Geometry check sheet. Reference: the model listing, model coordinates, mm. A direction names the side the tool comes from. Coordinates: 2 decimals unless noted, no trailing zeros. Order: outer loops, then holes, each group sorted by start corner. A loop starts at its lowest first (then second) coordinate and runs counter-clockwise, first axis right, second up. Notation, with made-up numbers: (8.5, -35.75) - (49.5, -35.75) arc R22 cw to (49.5, -13.75) - close; hole circle Ø11 at (75.5, -6.75). An arc over 180 degrees is marked (long way). Return JSON: item names as keys, results as strings. Group by question number.
Item 1: Section check C-C on y = 10. Enter the section's corners in (x, z) (3 decimals).
Item 2: Draft check along X on faces 1 (the flat face through (6, -14, 6.35)), 2 (the flat face through (6, -16.5, 3)), 3 (the cylindrical face through (-0.08, -32.25, 6.37)), 4 (the flat face through (9.157, 15.049, 3.87)). Enter one of: pulls with the +X half, pulls with the -X half, needs draft (parallel to the pull), parting line crosses it, or undercut.
Item 3: Gauge pin test, flat ends, axial feed: pin 1 (1.5 mm diameter, centred on y = -5.5, z = 2, fed in from +X) (3 decimals); pin 2 (1.9 mm diameter, centred on x = -4, y = -15, fed in from -Z) (3 decimals); pin 3 (1.5 mm diameter, centred on y = -14.5, z = 4, fed in from -X); pin 4 (8.5 mm diameter, centred on x = -2, y = -28.5, fed in from -Z). Record the tip position at first contact, or that the pin passes through.
Item 4: Section check D-D on y = -15. Enter the section's corners in (x, z) (3 decimals), then the cut area to 3 significant figures.
Item 5: Scan lines: probe 1 along Y at (x, z) = (7, 7.5); probe 2 along Y at (x, z) = (-4, 6); probe 3 along Y at (x, z) = (-1.75, 7). Record each from-to range of solid material in increasing order.
Item 6: Tool access check on faces 5 (the flat face through (6, 14, 6.35)), 6 (the flat face through (9, 11.5, 3)), 7 (the flat face through (1, -19.806, 6)), 8 (the flat face through (-1, -24, 4.85)), 9 (the flat face through (-6.641, -21, 6)). Record the directions out of +Z, -Z, +X, -X, +Y, -Y that give a thin tool (end or side, any length) a straight path to the whole face; none if there is none.
Item 7: Section check A-A on y = -8. Enter the section's corners in (x, z) (3 decimals), then the cut area to 3 significant figures.
Item 8: Section check B-B on x = 2.25. Enter the section's corners in (y, z).
from build123d import *

# Parameters (mm, degrees)
PAD_DEPTH       = 6.35
SKETCH001_W     = 19.26
SKETCH001_H     = 23
PAD001_DEPTH    = 1.5
SKETCH003_R     = 1.58
POCKET_DEPTH    = 98.88341
SKETCH002_W     = 4.4
SKETCH002_H     = 3.6
POCKET001_DEPTH = 14.106
FILLET_R        = 7
FILLET001_R     = 0.5
SKETCH004_R     = 1.58
PAD002_DEPTH    = 3


with BuildPart() as part:
    # Sketch → Pad (new body)
    with BuildSketch(Plane.XY):
        Polygon((4.355, -11.5), (-12.105, -11.5), (-12.105, 11.5), (4.355, 11.5), (4.355, 16.5), (7.155, 16.5), (7.155, 11.5), (11.215, 11.5), (7.155, 18.5), (-14.105, 18.5), (-14.105, -18.5), (7.155, -18.5), (11.215, -11.5), (7.155, -11.5), (7.155, -16.5), (4.355, -16.5), align=None)
    extrude(amount=PAD_DEPTH)

    # Sketch001 → Pad001 (join)
    with BuildSketch(Plane.XY.offset(6.35)):
        Polygon((-14.105, 0), (-14.105, 18.5), (7.155, 18.5), (11.215, 11.5), (11.215, -11.5), (7.155, -18.5), (-14.105, -18.5), align=None)
        with Locations((-2.475, 0)):
            Rectangle(SKETCH001_W, SKETCH001_H, mode=Mode.SUBTRACT)
    extrude(amount=PAD001_DEPTH)

    # Sketch003 → Pocket (cut, through all)
    with BuildSketch(Plane.XY):
        with Locations((-4, 15)):
            Circle(SKETCH003_R)
    pocket = extrude(amount=POCKET_DEPTH, mode=Mode.SUBTRACT)

    # Mirrored: Pocket across Sketch003 H_Axis
    add(pocket.mirror(Plane.ZX), mode=Mode.SUBTRACT)

    # Sketch002 → Pocket001 (cut, through all)
    with BuildSketch(Plane.YZ):
        with Locations((9.3, 1.8)):
            Rectangle(SKETCH002_W, SKETCH002_H)
    extrude(amount=-POCKET001_DEPTH, mode=Mode.SUBTRACT)

    # Fillet
    fillet_edges = [part.edges().sort_by_distance(p)[0] for p in [
        (-14.105, -18.5, 3.175),
        (-14.105, 18.5, 3.175),
    ]]
    fillet(fillet_edges, radius=FILLET_R)

    # Fillet001
    fillet001_edges = [part.edges().sort_by_distance(p)[0] for p in [
        (-13.105, 7.1, 0),
        (-13.105, 7.1, 3.6),
        (-13.105, 11.5, 3.6),
        (7.155, 14, 0),
        (5.755, 16.5, 0),
        (4.355, 14, 0),
        (7.155, -14, 0),
        (5.755, -16.5, 0),
        (4.355, -14, 0),
        (-5.58, -15, 0),
        (-5.58, 15, 0),
    ]]
    fillet(fillet001_edges, radius=FILLET001_R)

    # Sketch004 → Pad002 (join)
    with BuildSketch(Plane.XY.offset(7.85)):
        with BuildLine():
            Line((-6.6411, -18.5), (3.75, -18.5))
            Line((3.75, -18.5), (3.75, -28.5))
            ThreePointArc((-3.75, -28.5), (0, -32.25), (3.75, -28.5))
            Line((-3.75, -28.5), (-6.6411, -23.41))
            Line((-6.6411, -23.41), (-6.6411, -18.5))
        make_face()
        with Locations((0, -28.5)):
            Circle(SKETCH004_R, mode=Mode.SUBTRACT)
        with Locations((-3.75, -21.5)):
            Circle(SKETCH004_R, mode=Mode.SUBTRACT)
        Polygon((2.788238, -19.805846), (0, -19.805846), (-0.638352, -24.059963), (-3.75, -24.893727), (-3.75, -26.170431), (0, -25.165621), (0.612686, -21.08255), (2.788238, -21.08255), align=None, mode=Mode.SUBTRACT)
    extrude(amount=-PAD002_DEPTH)


solid = part.part
Computed:
{
 "1": {"outline": "(-14.105, 3.6) - (-12.105, 3.6) - (-12.105, 7.85) - (-14.105, 7.85) - close; (7.155, 6.35) - (11.215, 6.35) - (11.215, 7.85) - (7.155, 7.85) - close"},
 "2": {"face 1": "undercut", "face 2": "undercut", "face 3": "parting line crosses it", "face 4": "pulls with the +X half"},
 "3": {"pin 1": "stops at x = -12.105", "pin 2": "passes through", "pin 3": "stops at x = -13.73", "pin 4": "stops at z = 4.85"},
 "4": {"outline": "(-13.167, 0) - (-6.08, 0) arc R0.5 ccw to (-5.58, 0.5) - (-5.58, 7.85) - (-13.167, 7.85) - close; (-2.42, 0.5) arc R0.5 ccw to (-1.92, 0) - (3.855, 0) arc R0.5 ccw to (4.355, 0.5) - (4.355, 6.35) - (7.155, 6.35) - (7.155, 0.5) arc R0.5 ccw to (7.655, 0) - (9.185, 0) - (9.185, 7.85) - (-2.42, 7.85) - close", "area": "133 mm²"},
 "5": {"probe 1": "y = -18.5 to -11.5, 11.5 to 18.5", "probe 2": "y = -28.06 to -23.06, -19.94 to -16.58, -13.42 to -11.5, 11.5 to 13.42, 16.58 to 18.5", "probe 3": "y = -31.82 to -25.63, -24.36 to -11.5, 11.5 to 18.5"},
 "6": {"face 5": "-Z", "face 6": "-Z, +X", "face 7": "+Z, -Z", "face 8": "-Z, +X, -X, -Y", "face 9": "+Z, -Z, -X, -Y"},
 "7": {"outline": "(-14.105, 0) - (-12.105, 0) - (-12.105, 7.85) - (-14.105, 7.85) - close; (7.155, 6.35) - (11.215, 6.35) - (11.215, 7.85) - (7.155, 7.85) - close", "area": "21.8 mm²"},
 "8": {"outline": "(-31.5, 4.85) - (-21.08, 4.85) - (-21.08, 7.85) - (-31.5, 7.85) - close; (-19.81, 4.85) - (-18.5, 4.85) - (-18.5, 0) - (-11.5, 0) - (-11.5, 7.85) - (-19.81, 7.85) - close; (11.5, 0) - (18.5, 0) - (18.5, 7.85) - (11.5, 7.85) - close"}
}
